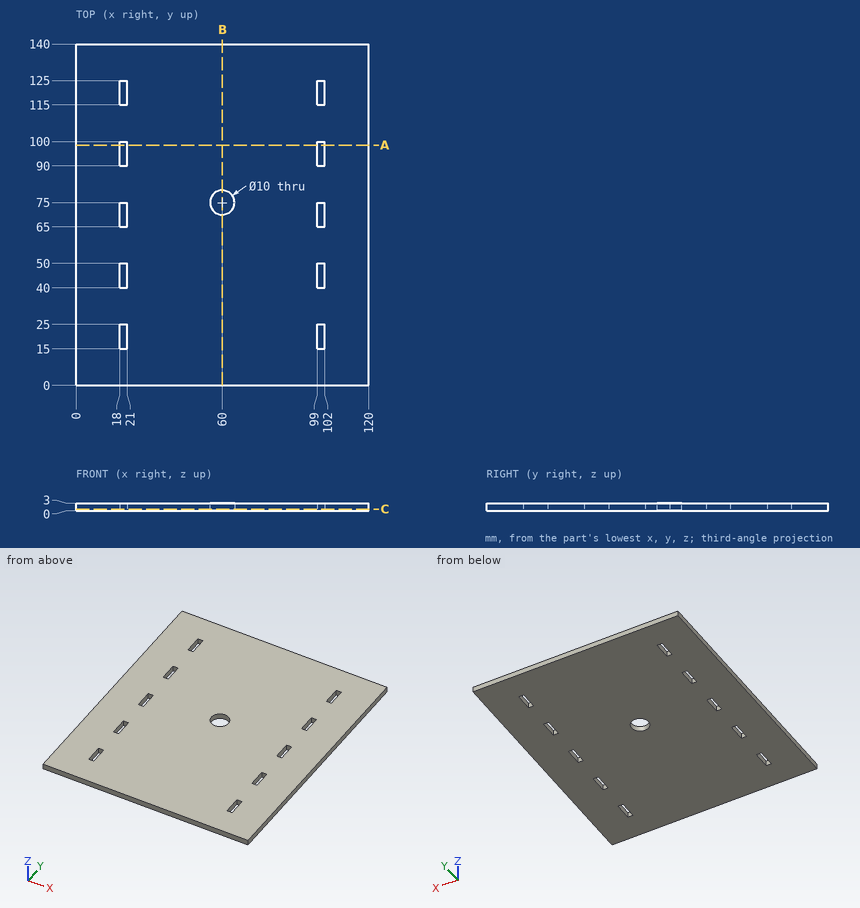
Geometry check sheet. Reference: drawing and pictorial views, mm from the part's lowest x, y, z. Give positions to 0.01 mm unless a question says otherwise; leave off trailing zeros. Loops run counter-clockwise (first coordinate to the right, second up) from the corner with the lowest first, then second, coordinate; pieces in that order, holes last. Notation, with made-up numbers: M 69.25,-24 L 79.25,-24 A18 cw 79.25,-4 Z; hole C 50,-29 d10. An arc over 180 degrees is marked long. Use a Markdown table: item, result. Add a question column.
Q1. Sectioned sample at B-B, the plane x = 60. Record the cut outline in (y, z), then the cut area to 3 significant figures.
Q2. Sectioned sample at C-C, the plane z = 0.6. Give the number of separate pieces and of enclosed holes in the cut face, then the cut area to 3 significant figures.
Q3. Scan lines: line 1 along X through (y, z) = (94, 0.25); line 2 along Y through (x, z) = (60, 1.15). Record each from-to range of solid material in increasing order. Write a range as [from, to].
Q4. Sectioned sample at A-A, the plane y = 98.5. Record the cut outline in (x, z), then the cut area to 3 significant figures.
Verdict:
| question | item | result |
|---|---|---|
| 1 | outline | M 0,0 L 70,0 L 70,3 L 0,3 Z; M 80,0 L 140,0 L 140,3 L 80,3 Z |
| 1 | area | 390 mm^2 |
| 2 | separate pieces | 1 |
| 2 | enclosed holes | 11 |
| 2 | area | 16,400 mm^2 |
| 3 | line 1 | [0, 18], [21, 99], [102, 120] |
| 3 | line 2 | [0, 70], [80, 140] |
| 4 | outline | M 0,0 L 18,0 L 18,3 L 0,3 Z; M 21,0 L 99,0 L 99,3 L 21,3 Z; M 102,0 L 120,0 L 120,3 L 102,3 Z |
| 4 | area | 342 mm^2 |
